Can you work these out from the model? Positions are in its coordinate system, mm. Face numbers are marked on the shaded views. A direction names the side the tool comes from. Coordinates: 2 decimals unless noted, no trailing zeros. Order: outer loops, then holes, each group sorted by start corner. A loop starts at its lowest first (then second) coordinate and runs counter-clockwise, first axis right, second up.
```python
from build123d import *

# Parameters (mm, degrees)
F1_DEPTH = 8
F2_R     = 1.5
F3_DEPTH = 12.5
F4_SIZE  = 1.99999
F5_R     = 3
F6_DEPTH = 4
F8_DEPTH = 2


# Not quite as in the source:
# - a fillet or chamfer is up to 0.001 mm smaller than in the source, because OpenCascade refuses the exact size


with BuildPart() as f1:
    # F0 (on Front) → F1 (new body)
    with BuildSketch(Plane.XZ):
        Polygon((5.1, 5.1), (5.1, -5.1), (-5.1, -5.1), (-5.1, 5.1), (-4.1, 5.1), (-1.1, 5.1), (-1.1, 8.1), (-1.1, 17.1), (-4.1, 17.1), (-4.1, 8.1), (-5.1, 8.1), (-8.1, 8.1), (-8.1, -8.1), (8.1, -8.1), (8.1, 8.1), (2.9, 8.1), (2.9, 17.1), (-0.1, 17.1), (-0.1, 8.1), (-0.1, 5.1), align=None)
    extrude(amount=F1_DEPTH)

    # F2 (on face) → F3 (cut, symmetric)
    with BuildSketch(Plane.YZ.offset(-1.1)):
        with Locations((-5, 11.6)):
            Circle(F2_R)
    extrude(amount=F3_DEPTH, both=True, mode=Mode.SUBTRACT)

    # F4 (size 2 in the source; OpenCascade refuses exactly that, so slightly less here)
    f4_edges = [f1.edges().sort_by_distance(p)[0] for p in [
        (2.9, -4, 8.1),
    ]]
    chamfer(f4_edges, length=F4_SIZE)

    # F5 (on face) → F6 (cut)
    with BuildSketch(Plane.YZ.offset(2.9)):
        with Locations((-5, 11.6)):
            Circle(F5_R)
    extrude(amount=F6_DEPTH, mode=Mode.SUBTRACT)

    # F7 (on face) → F8 (join)
    with BuildSketch(Plane(origin=(0, 0, 0), x_dir=(-1, 0, 0), z_dir=(0, 1, 0))):
        Polygon((4.1, 8.1), (8.1, 8.1), (4.1, 12.6), align=None)
    extrude(amount=-F8_DEPTH)


solid = f1.part
```
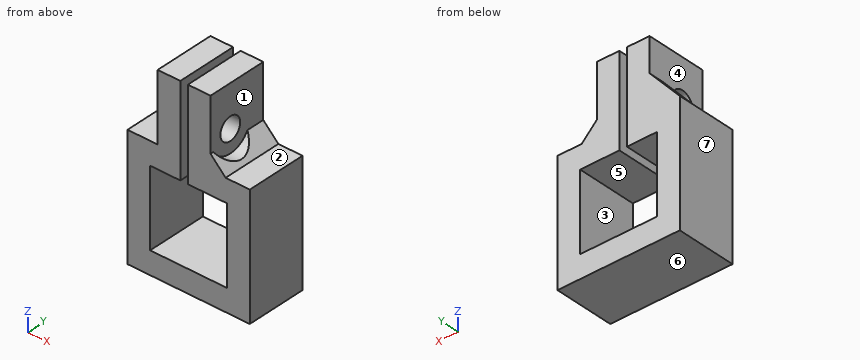
1. On a 3-axis mill with a long thin cutter (end or side, diameter ignored), from which of +Z, -Z, +X, -X, +Y, -Y can I reach the whole of each face in a straight line? I mean the marked faces 1, 2, 3 and 4. Say none if no direction works.
Completed:
face 1: +Z, +X
face 2: +Z, +X, +Y, -Y
face 3: +Y, -Y
face 4: +Z, -X, -Y
2. I'm going to push flat-ended pins straight in: pin 1 (2.5 mm diameter, centred on x = 7, y = -4.5, fed in from +Z); pin 2 (2.5 mm diameter, centred on y = -2.5, z = 12.5, fed in from +X). Where does each tip first touch, or does it pass through?
Completed:
pin 1: stops at z = 8.1
pin 2: stops at x = 2.9
3. Please list where these lines run through material, in increasing order: probe 1 along Z at (x, y) = (0.65, -5); probe 2 along X at (y, z) = (-1, 1.75); probe 3 along X at (y, z) = (-3.75, 7).
Completed:
probe 1: z = -8.1 to -5.1, 5.1 to 10.1, 13.1 to 17.1
probe 2: x = -8.1 to -5.1, 5.1 to 8.1
probe 3: x = -8.1 to -1.1, -0.1 to 8.1
4. Imagine slicing it at D-D on x = -5.75. Please give me the cut outline in (y, z).
Completed:
outline: (-8, -8.1) - (0, -8.1) - (0, 10.74) - (-2, 10.74) - (-2, 8.1) - (-8, 8.1) - close
5. Imagine slicing it at A-A on x = 2.5. Please give me the cut outline in (y, z).
Completed:
outline: (-8, -8.1) - (0, -8.1) - (0, -5.1) - (-8, -5.1) - close; (-8, 5.1) - (0, 5.1) - (0, 17.1) - (-8, 17.1) - close; hole circle Ø3 at (-5, 11.6)
6. Thinking about a two-plate mould opening in Z: for the marked faces 5, 6 and 7, which applies, pulls with the +Z half, pulls with the -Z half, needs draft (parallel to the pull), parting line crosses it, or undercut?
Completed:
face 5: undercut
face 6: pulls with the -Z half
face 7: needs draft
7. Imagine slicing it at C-C on z = 11.6. Please give me the cut outline in (x, y), then the cut area to 3 significant figures.
Completed:
outline: (-4.99, -2) - (-4.1, -2) - (-4.1, -3.5) - (-1.1, -3.5) - (-1.1, 0) - (-4.99, 0) - close; (-4.1, -8) - (-1.1, -8) - (-1.1, -6.5) - (-4.1, -6.5) - close; (-0.1, -8) - (2.9, -8) - (2.9, -6.5) - (-0.1, -6.5) - close; (-0.1, -3.5) - (2.9, -3.5) - (2.9, 0) - (-0.1, 0) - close
area: 31.8 mm2
8. Imagine slicing it at B-B on y = -5. Please give me the cut outline in (x, z), then the cut area to 3 significant figures.
Completed:
outline: (-8.1, -8.1) - (8.1, -8.1) - (8.1, 8.1) - (4.9, 8.1) - (4.4, 8.6) - (2.9, 8.6) - (2.9, 10.1) - (-0.1, 10.1) - (-0.1, 5.1) - (5.1, 5.1) - (5.1, -5.1) - (-5.1, -5.1) - (-5.1, 5.1) - (-1.1, 5.1) - (-1.1, 10.1) - (-4.1, 10.1) - (-4.1, 8.1) - (-8.1, 8.1) - close; (-4.1, 13.1) - (-1.1, 13.1) - (-1.1, 17.1) - (-4.1, 17.1) - close; (-0.1, 13.1) - (2.9, 13.1) - (2.9, 17.1) - (-0.1, 17.1) - close
area: 192 mm2
